The listing builds one solid part. Answer for the finished solid, in the listing's coordinates (mm). Face numbers are marked on the shaded views. A direction names the side the tool comes from. Give positions to 0.01 mm unless a question says otherwise; leave off trailing zeros. Order: outer loops, then holes, each group sorted by start corner. A loop starts at its lowest first (then second) coordinate and runs counter-clockwise, first axis right, second up. Notation, with made-up numbers: (73, 21.25) - (106, 21.25) arc R17 cw to (106, 44.25) - close; hole circle Ø7 at (27, -4.75). An arc over 180 degrees is marked (long way). Use a Markdown table: item, result. Add a question column.
1) The mould has two halves that part along Y. Classify the marked faces 5, 6 and 7: released by +Y, released by -Y, zero draft, split by the parting line, or undercut.
2) Flat-ended cylindrical pins translate along their axes: pin 1 (17 mm diameter, centred on x = -6, z = 24, fed in from -Y); pin 2 (8 mm diameter, centred on y = 54, z = 18, fed in from -X); pin 3 (9.5 mm diameter, centred on x = -29, z = 14.5, fed in from +Y); pin 4 (7.5 mm diameter, centred on y = -14.05, z = 17, fed in from -X). Find the tip coordinate at first contact, or state that the pin passes through.
3) Find section B-B, the plane z = 17. State how many separate pieces and enclosed holes the cut face has, plus the area to 3 significant figures.
4) Find section C-C, the plane y = -14.05. Determine the outline of the cut face in (x, z), plus the area to 3 significant figures.
5) Straight lines are drawn through the part: line 1 (Z direction, x = -22.15, y = -14.05); line 2 (X direction, y = -11, z = 8); line 3 (X direction, y = 28.5, z = 4). For each, find the intervals that lie inside material, in ascending order.
6) Find section D-D, the plane x = 35.5. Determine the outline of the cut face in (y, z), plus the area to 3 significant figures.
7) For the marked faces 1, 2, 3 and 4, determine the directions among +Z, -Z, +X, -X, +Y, -Y from which every point of the face is accessible in a straight line to the end or side of a thin tool.
8) Find section A-A, the plane y = 18. Determine the outline of the cut face in (x, z).
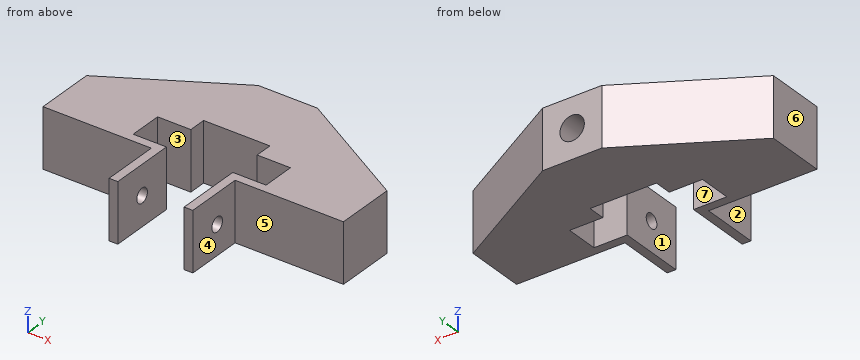
from build123d import *

# Parameters (mm, degrees)
BOSS_EXTRUDE1_DEPTH = 34
SKETCH2_R           = 7
CUT_EXTRUDE1_DEPTH  = 35
SKETCH3_R           = 4.1656
CUT_EXTRUDE2_DEPTH  = 138.185886126


with BuildPart() as part:
    # Sketch1 → Boss-Extrude1 (new body)
    with BuildSketch(Plane.XY):
        Polygon((-86.282032303, 0), (-24.05, 0), (-24.05, -33.1), (-19.05, -33.1), (-19.05, 5), (-38.15, 5), (-38.15, 24.1), (-19.05, 24.1), (-19.05, 34.1), (19.05, 34.1), (19.05, 24.1), (38.15, 24.1), (38.15, 5), (19.05, 5), (19.05, -33.1), (24.05, -33.1), (24.05, 0), (86.282032303, 0), (86.282032303, 34.1), (17, 74.1), (-17, 74.1), (-86.282032303, 34.1), align=None)
    extrude(amount=BOSS_EXTRUDE1_DEPTH)

    # Sketch2 → Cut-Extrude1 (cut)
    with BuildSketch(Plane(origin=(0, 74.1, 0), x_dir=(1, 0, 0), z_dir=(0, 1, 0))):
        with Locations(Location((0, -17, 0), (0, 0, 270))):
            Circle(SKETCH2_R)
    extrude(amount=-CUT_EXTRUDE1_DEPTH, mode=Mode.SUBTRACT)

    # Sketch3 → Cut-Extrude2 (cut, through all)
    with BuildSketch(Plane(origin=(24.05, 0, 0), x_dir=(0, 0, -1), z_dir=(1, 0, 0))):
        with Locations(Location((-17, -14.05, 0), (0, 0, 90))):
            Circle(SKETCH3_R)
    extrude(amount=-CUT_EXTRUDE2_DEPTH, mode=Mode.SUBTRACT)


solid = part.part
The answers:
| question | item | result |
|---|---|---|
| 1 | face 5 | released by -Y |
| 1 | face 6 | zero draft |
| 1 | face 7 | undercut |
| 2 | pin 1 | y = 34.1 |
| 2 | pin 2 | x = -58.74 |
| 2 | pin 3 | y = 69.91 |
| 2 | pin 4 | through |
| 3 | separate pieces | 3 |
| 3 | enclosed holes | 0 |
| 3 | area | 7,740 mm2 |
| 4 | outline | (-24.05, 0) - (-19.05, 0) - (-19.05, 12.83) - (-24.05, 12.83) - close; (-24.05, 21.17) - (-19.05, 21.17) - (-19.05, 34) - (-24.05, 34) - close; (19.05, 0) - (24.05, 0) - (24.05, 12.83) - (19.05, 12.83) - close; (19.05, 21.17) - (24.05, 21.17) - (24.05, 34) - (19.05, 34) - close |
| 4 | area | 257 mm2 |
| 5 | line 1 | 0 to 12.83, 21.17 to 34 |
| 5 | line 2 | -24.05 to -19.05, 19.05 to 24.05 |
| 5 | line 3 | -86.28 to -19.05, 19.05 to 86.28 |
| 6 | outline | (0, 0) - (5, 0) - (5, 34) - (0, 34) - close; (24.1, 0) - (63.42, 0) - (63.42, 34) - (24.1, 34) - close |
| 6 | area | 1,510 mm2 |
| 7 | face 1 | +Z, -Z, -Y |
| 7 | face 2 | +Z, -Z, -X, -Y |
| 7 | face 3 | +Z, -Z |
| 7 | face 4 | +Z, -Z, +X, -Y |
| 8 | outline | (-86.28, 0) - (-38.15, 0) - (-38.15, 34) - (-86.28, 34) - close; (38.15, 0) - (86.28, 0) - (86.28, 34) - (38.15, 34) - close |
